Study the drawing (mm; zero at the part's minimum x, y, z) and answer. A direction names the side the tool comes from. Round coordinates to 2 decimals unless told otherwise and drop trailing zeros. Write each loop counter-clockwise with the first axis right and the second up, starting at its lowest first coordinate (ties: lowest second). Pieces come first, ordered by that corner, then holes.
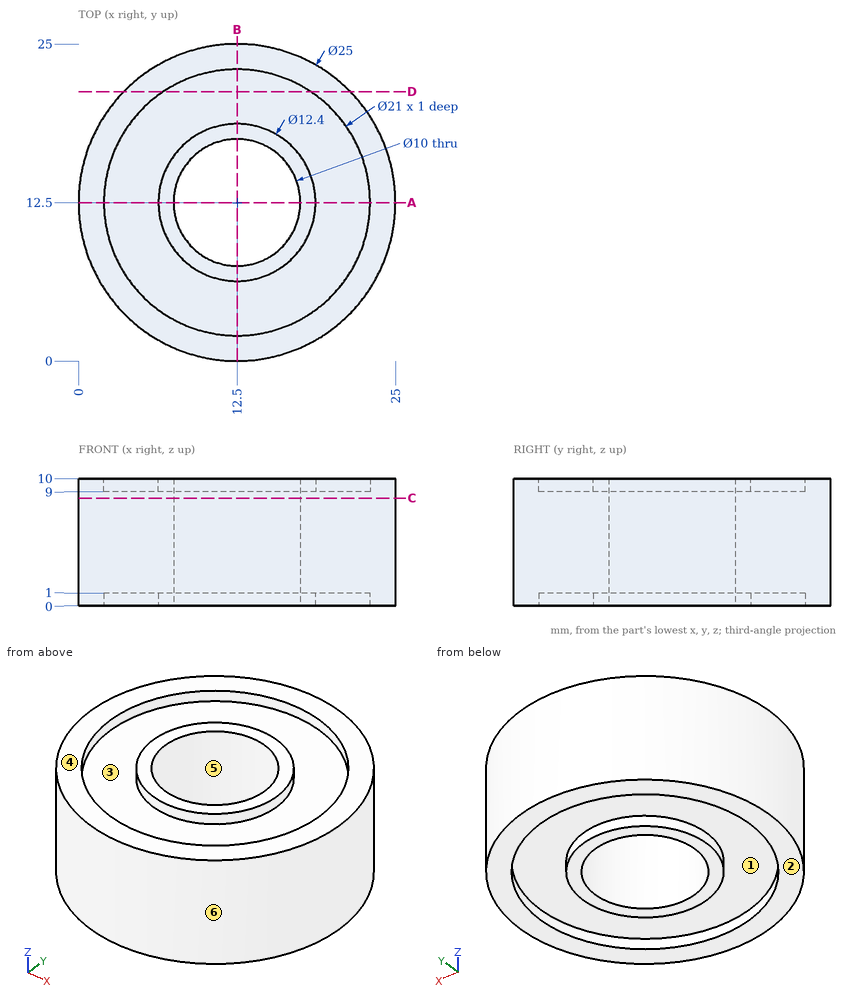
1. Section A-A on y = 12.5 is taken. Determine the outline of the cut face in (x, z).
Geometry says:
outline: (0, 0) - (2, 0) - (2, 1) - (6.3, 1) - (6.3, 0) - (7.5, 0) - (7.5, 10) - (6.3, 10) - (6.3, 9) - (2, 9) - (2, 10) - (0, 10) - close; (17.5, 0) - (18.7, 0) - (18.7, 1) - (23, 1) - (23, 0) - (25, 0) - (25, 10) - (23, 10) - (23, 9) - (18.7, 9) - (18.7, 10) - (17.5, 10) - close
2. A tool of negligible diameter and unlimited length cuts with its end or side. For the marked faces 1, 2 and 3, from which of +Z, -Z, +X, -X, +Y, -Y can it reach the whole face along a straight path? Write none if from no direction.
Geometry says:
face 1: -Z
face 2: -Z, +X, -X, +Y, -Y
face 3: +Z
3. Given pin 1 (6 mm diameter, centred on x = 12.5, y = 12.5, fed in from -Z); pin 2 (1.5 mm diameter, centred on y = 7.5, z = 3, fed in from +X); pin 3 (1.5 mm diameter, centred on x = 13.5, z = 7.5, fed in from +Y); pin 4 (1 mm diameter, centred on x = 21.5, y = 10, fed in from -Z), each flat-ended and moving along its own axis, determine where each tip first touches the part or whether it passes through.
Geometry says:
pin 1: passes through
pin 2: stops at x = 24.26
pin 3: stops at y = 25
pin 4: stops at z = 1
4. Section C-C on z = 8.5 is taken. Determine the outline of the cut face in (x, y).
Geometry says:
outline: circle Ø25 at (12.5, 12.5); hole circle Ø10 at (12.5, 12.5)
5. Section D-D on y = 21.25 is taken. Determine the outline of the cut face in (x, z), plus the area to 3 significant figures.
Geometry says:
outline: (3.57, 0) - (6.7, 0) - (6.7, 1) - (18.3, 1) - (18.3, 0) - (21.43, 0) - (21.43, 10) - (18.3, 10) - (18.3, 9) - (6.7, 9) - (6.7, 10) - (3.57, 10) - close
area: 155 mm2
6. For a pull along X with two mould halves and no side action, classify the marked faces 4, 5 and 6 as released by +X, released by -X, zero draft, split by the parting line, or undercut.
Geometry says:
face 4: zero draft
face 5: undercut
face 6: split by the parting line
7. Straight lines are drawn through the part: line 1 along Y through (x, z) = (12.5, 9.8); line 2 along Y through (x, z) = (14, 0.5); line 3 along Z through (x, y) = (16.5, 4.25). For each, find the intervals that lie inside material, in ascending order.
Geometry says:
line 1: y = 0 to 2, 6.3 to 7.5, 17.5 to 18.7, 23 to 25
line 2: y = 0.09 to 2.11, 6.48 to 7.73, 17.27 to 18.52, 22.89 to 24.91
line 3: z = 1 to 9
